Can you work these out from the drawing? Everything is in mm from the part's minimum corner. Give positions to 0.01 mm unless a question says otherwise; leave off trailing zeros. Write each loop counter-clockwise with the first axis right and the second up, starting at its lowest first coordinate (ties: lowest second). Pieces come first, ordered by that corner, then holes. Notation, with made-up numbers: (-4.75, 85) - (11.25, 85) arc R15 cw to (11.25, 101) - close; hole circle Ø7 at (63.25, -31.75). An arc over 180 degrees is marked (long way). Return JSON: item names as keys, results as strings. Group by question number.
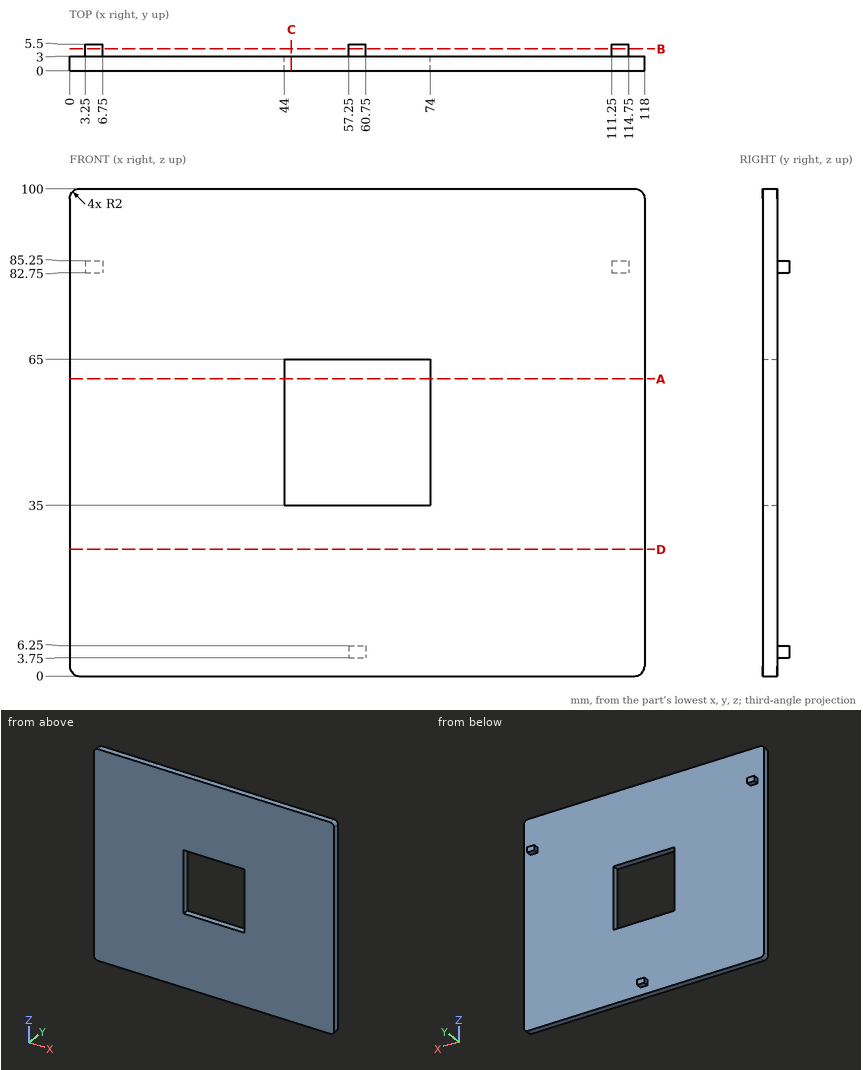
1) I need wall thicknesses on line 1 along Z through (x, y) = (71.5, 2.2); line 2 along Y through (x, z) = (72, 81.5); line 3 along Z through (x, y) = (113, 5.05). Which ranges of each line are inside material? Lowest first, please.
2) Imagine slicing it at C-C, the plane x = 45.5. Write out the boundary of the cut face in (y, z), and give its area (3 significant figures).
3) Imagine slicing it at D-D, the plane z = 26. Write out the boundary of the cut face in (x, y).
4) Imagine slicing it at A-A, the plane z = 61. Write out the boundary of the cut face in (x, y).
5) Imagine slicing it at B-B, the plane y = 4.5. Write out the boundary of the cut face in (x, z), and give its area (4 significant figures).
6) Will these pins go through, and if not, where does the flat tip stop? pin 1 Ø0.8 at (x, y) = (113, 3.5) entering from -Z; pin 2 Ø1.2 at (y, z) = (4, 84.5) entering from +X; pin 3 Ø8 at (x, z) = (18, 40.5) entering from +Y.
Resolved:
{
 "1": {"line 1": "0 to 35, 65 to 100", "line 2": "0 to 3", "line 3": "82.75 to 85.25"},
 "2": {"outline": "(0, 0) - (3, 0) - (3, 35) - (0, 35) - close; (0, 65) - (3, 65) - (3, 100) - (0, 100) - close", "area": "210 mm^2"},
 "3": {"outline": "(0, 0) - (118, 0) - (118, 3) - (0, 3) - close"},
 "4": {"outline": "(0, 0) - (44, 0) - (44, 3) - (0, 3) - close; (74, 0) - (118, 0) - (118, 3) - (74, 3) - close"},
 "5": {"outline": "(3.25, 82.75) - (6.75, 82.75) - (6.75, 85.25) - (3.25, 85.25) - close; (57.25, 3.75) - (60.75, 3.75) - (60.75, 6.25) - (57.25, 6.25) - close; (111.25, 82.75) - (114.75, 82.75) - (114.75, 85.25) - (111.25, 85.25) - close", "area": "26.25 mm^2"},
 "6": {"pin 1": "z = 82.75", "pin 2": "x = 114.75", "pin 3": "y = 3"}
}
